```python
from build123d import *

# Parameters (mm, degrees)
SKETCH1_W                              = 100
SKETCH1_H                              = 170
BOSS_EXTRUDE1_DEPTH                    = 40
F_1_8_27_NPSM_TAPPED_HOLE1_D           = 9.0932
F_1_8_27_NPSM_TAPPED_HOLE1_DEPTH       = 22.987
F_1_8_27_NPSM_TAPPED_HOLE1_CSINK_D     = 10.1338
F_1_8_27_NPSM_TAPPED_HOLE1_CSINK_ANGLE = 90
F_1_8_27_NPSM_TAPPED_HOLE1_TIP         = 2.73187289
SKETCH11_W                             = 45.5
SKETCH11_H                             = 105.5
CUT_EXTRUDE3_DEPTH                     = 35
CUT_EXTRUDE4_DEPTH                     = 35
SKETCH13_W                             = 22.5
SKETCH13_H                             = 15
CUT_EXTRUDE5_DEPTH                     = 35
FILLET1_R                              = 5
FILLET2_R                              = 5
M3X0_5_TAPPED_HOLE1_D                  = 2.5
M3X0_5_TAPPED_HOLE1_DEPTH              = 7.5
M3X0_5_TAPPED_HOLE1_CSINK_D            = 3.05
M3X0_5_TAPPED_HOLE1_CSINK_ANGLE        = 90
M3X0_5_TAPPED_HOLE1_TIP                = 0.751075774
FILLET3_R                              = 5


with BuildPart() as part:
    # Sketch1 → Boss-Extrude1 (new body)
    with BuildSketch(Plane.XY):
        with Locations((50, 85)):
            Rectangle(SKETCH1_W, SKETCH1_H)
    extrude(amount=BOSS_EXTRUDE1_DEPTH)

    # 1/8-27 NPSM Tapped Hole1
    with Locations(Plane(origin=(0, 170, 0), x_dir=(1, 0, 0), z_dir=(0, 1, 0))):
        with Locations((37.5, -20), (62.5, -20)):
            CounterSinkHole(F_1_8_27_NPSM_TAPPED_HOLE1_D / 2, F_1_8_27_NPSM_TAPPED_HOLE1_CSINK_D / 2, depth=F_1_8_27_NPSM_TAPPED_HOLE1_DEPTH, counter_sink_angle=F_1_8_27_NPSM_TAPPED_HOLE1_CSINK_ANGLE)
            with Locations((0, 0, -(F_1_8_27_NPSM_TAPPED_HOLE1_DEPTH + F_1_8_27_NPSM_TAPPED_HOLE1_TIP / 2))):  # 118° drill point
                Cone(0, F_1_8_27_NPSM_TAPPED_HOLE1_D / 2, F_1_8_27_NPSM_TAPPED_HOLE1_TIP, mode=Mode.SUBTRACT)

    # Sketch11 → Cut-Extrude3 (cut)
    with BuildSketch(Plane.XY.offset(40)):
        with Locations((50, 85)):
            Rectangle(SKETCH11_W, SKETCH11_H)
    extrude(amount=-CUT_EXTRUDE3_DEPTH, mode=Mode.SUBTRACT)

    # Sketch12 → Cut-Extrude4 (cut)
    with BuildSketch(Plane(origin=(0, 0, 0), x_dir=(-1, 0, 0), z_dir=(0, 0, -1))):
        Polygon((-90, 160), (-75, 160), (-75, 25), (-25, 25), (-25, 160), (-10, 160), (-10, 10), (-25, 10), (-75, 10), (-90, 10), align=None)
    extrude(amount=-CUT_EXTRUDE4_DEPTH, mode=Mode.SUBTRACT)

    # Sketch13 → Cut-Extrude5 (cut)
    with BuildSketch(Plane(origin=(0, 0, 0), x_dir=(-1, 0, 0), z_dir=(0, 0, -1))):
        with Locations((-63.75, 152.5)):
            Rectangle(SKETCH13_W, SKETCH13_H)
        with Locations((-36.25, 152.5)):
            Rectangle(SKETCH13_W, SKETCH13_H)
    extrude(amount=-CUT_EXTRUDE5_DEPTH, mode=Mode.SUBTRACT)

    # Fillet1
    fillet1_edges = [part.edges().sort_by_distance(p)[0] for p in [
        (90, 10, 17.5),
        (90, 160, 17.5),
        (75, 25, 17.5),
        (25, 25, 17.5),
        (10, 160, 17.5),
        (10, 10, 17.5),
        (52.5, 145, 17.5),
        (75, 145, 17.5),
        (52.5, 160, 17.5),
        (25, 145, 17.5),
        (47.5, 160, 17.5),
        (47.5, 145, 17.5),
    ]]
    fillet(fillet1_edges, radius=FILLET1_R)

    # Fillet2
    fillet2_edges = [part.edges().sort_by_distance(p)[0] for p in [
        (27.25, 32.25, 22.5),
        (27.25, 137.75, 22.5),
        (72.75, 137.75, 22.5),
        (72.75, 32.25, 22.5),
    ]]
    fillet(fillet2_edges, radius=FILLET2_R)

    # M3x0.5 Tapped Hole1
    with Locations(Plane(origin=(0, 0, 0), x_dir=(-1, 0, 0), z_dir=(0, 0, -1))):
        with Locations((-95, 165), (-50, 165), (-5, 165), (-5, 85), (-5, 5), (-50, 5), (-95, 5), (-95, 85)):
            CounterSinkHole(M3X0_5_TAPPED_HOLE1_D / 2, M3X0_5_TAPPED_HOLE1_CSINK_D / 2, depth=M3X0_5_TAPPED_HOLE1_DEPTH, counter_sink_angle=M3X0_5_TAPPED_HOLE1_CSINK_ANGLE)
            with Locations((0, 0, -(M3X0_5_TAPPED_HOLE1_DEPTH + M3X0_5_TAPPED_HOLE1_TIP / 2))):  # 118° drill point
                Cone(0, M3X0_5_TAPPED_HOLE1_D / 2, M3X0_5_TAPPED_HOLE1_TIP, mode=Mode.SUBTRACT)

    # Fillet3
    fillet3_edges = [part.edges().sort_by_distance(p)[0] for p in [
        (0, 170, 20),
        (100, 170, 20),
        (100, 0, 20),
        (0, 0, 20),
    ]]
    fillet(fillet3_edges, radius=FILLET3_R)


solid = part.part
```
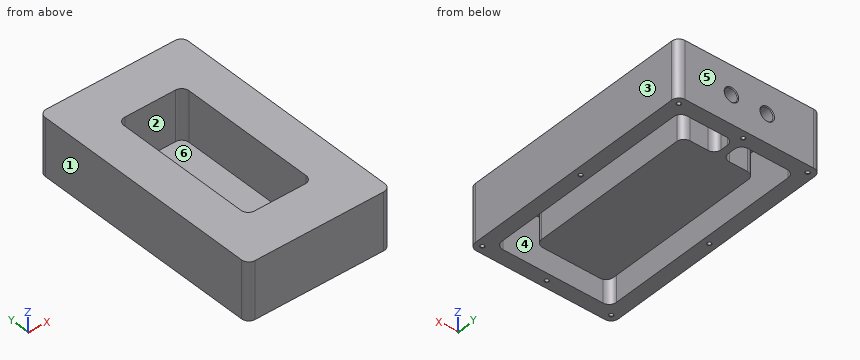
Input: part model. Units: mm. Frame: model coordinates. Face numbers are marked on the shaded views. A direction names the side the tool comes from. Round coordinates to 2 decimals unless told otherwise and drop trailing zeros. Loops run counter-clockwise (first coordinate to the right, second up) from the corner with the lowest first, then second, coordinate; pieces in that order, holes last. Notation, with made-up numbers: M 12,6.5 L 26,6.5 A8 cw 26,21.5 Z; hole C -6.75,0.25 d9. An arc over 180 degrees is marked long. Answer in a Markdown table with one row per item. Add a question column.
1. Section B-B (y = 23). Output: boundary loops of the cut face in (x, z), and give its area (3 significant figures).
2. Contact query for flat-ended pins moving along their axis: pin 1 (23 mm diameter, centred on x = 56, y = 91, fed in from +Z); pin 2 (5.5 mm diameter, centred on x = 37.5, z = 20, fed in from +Y); pin 3 (10 mm diameter, centred on x = 66, z = 19, fed in from +Y). Output: stop coordinate, or through.
3. Section D-D (y = 58.5). Output: boundary loops of the cut face in (x, z), and give its area (3 significant figures).
4. Section C-C (z = 10). Give the number of separate pieces and of enclosed holes in the cut face, and give its area (3 significant figures).
5. Set-up query: the marked faces 4, 5 and 6. Return all of +Z, -Z, +X, -X, +Y, -Y with unobstructed straight access to the full face (end or side cutting, diameter ignored); none if empty.
6. Section A-A (x = 18). Output: boundary loops of the cut face in (y, z).
7. Ray query, probe 1 along X at (y, z) = (165, 2.5); probe 2 along Y at (x, z) = (95, 4); probe 3 along Y at (x, z) = (34, 9.5). Return the intervals inside material, ascending.
8. Mould query, pull axis X, two halves, no side actions, for the marked faces 1, 2 and 3. Classes: released by +X, released by -X, zero draft, split by the parting line, or undercut.
Values follow:
| question | item | result |
|---|---|---|
| 1 | outline | M 0,0 L 10,0 L 10,35 L 90,35 L 90,0 L 100,0 L 100,40 L 0,40 Z |
| 1 | area | 1,200 mm^2 |
| 2 | pin 1 | z = 5 |
| 2 | pin 2 | y = 145 |
| 2 | pin 3 | y = 170 |
| 3 | outline | M 0,0 L 10,0 L 10,35 L 25,35 L 25,0 L 75,0 L 75,35 L 90,35 L 90,0 L 100,0 L 100,40 L 72.75,40 L 72.75,5 L 27.25,5 L 27.25,40 L 0,40 Z |
| 3 | area | 1,360 mm^2 |
| 4 | separate pieces | 1 |
| 4 | enclosed holes | 2 |
| 4 | area | 6,300 mm^2 |
| 5 | face 4 | -Z |
| 5 | face 5 | +Z, -Z, +X, -X, +Y |
| 5 | face 6 | +Z |
| 6 | outline | M 0,0 L 10,0 L 10,35 L 160,35 L 160,0 L 170,0 L 170,40 L 0,40 Z |
| 7 | probe 1 | 0 to 3.75, 6.25 to 48.75, 51.25 to 93.75, 96.25 to 100 |
| 7 | probe 2 | 0 to 3.75, 6.25 to 83.75, 86.25 to 163.75, 166.25 to 170 |
| 7 | probe 3 | 0 to 10, 25 to 32.25, 137.75 to 145, 160 to 170 |
| 8 | face 1 | released by -X |
| 8 | face 2 | undercut |
| 8 | face 3 | released by +X |
